```python
from build123d import *

# Parameters (mm, degrees)
SKETCH1_W           = 60
SKETCH1_H           = 35
SKETCH1_W_2         = 40.2
SKETCH1_H_2         = 20.2
BOSS_EXTRUDE1_DEPTH = 5
SKETCH2_W           = 60
SKETCH2_H           = 5
BOSS_EXTRUDE2_DEPTH = 29
SKETCH3_R           = 2
CUT_EXTRUDE1_DEPTH  = 10
SKETCH4_R           = 2
CUT_EXTRUDE2_DEPTH  = 48.451090489


with BuildPart() as part:
    # Sketch1 → Boss-Extrude1 (new body)
    with BuildSketch(Plane.XY):
        with Locations((-2.1, -1.998615043)):
            Rectangle(SKETCH1_W, SKETCH1_H)
        with Locations((-2.2, 0.601384957)):
            Rectangle(SKETCH1_W_2, SKETCH1_H_2, mode=Mode.SUBTRACT)
    extrude(amount=BOSS_EXTRUDE1_DEPTH)

    # Sketch2 → Boss-Extrude2 (add)
    with BuildSketch(Plane.XY.offset(5)):
        with Locations((-2.1, -16.998615043)):
            Rectangle(SKETCH2_W, SKETCH2_H)
    extrude(amount=BOSS_EXTRUDE2_DEPTH)

    # Sketch3 → Cut-Extrude1 (cut)
    with BuildSketch(Plane(origin=(0, -19.498615043, 0), x_dir=(-1, 0, 0), z_dir=(0, -1, 0))):
        with Locations(Location((17.1, -15, 0), (0, 0, 90))):
            Circle(SKETCH3_R)
        with Locations(Location((-12.9, -15, 0), (0, 0, 90))):
            Circle(SKETCH3_R)
    extrude(amount=-CUT_EXTRUDE1_DEPTH, mode=Mode.SUBTRACT)

    # Sketch4 → Cut-Extrude2 (cut, through all)
    with BuildSketch(Plane.XY.offset(5)):
        with Locations((21.9, 5.601384957)):
            Circle(SKETCH4_R)
        with Locations((21.9, -4.398615043)):
            Circle(SKETCH4_R)
        with Locations((-26.1, -4.398615043)):
            Circle(SKETCH4_R)
        with Locations((-26.1, 5.601384957)):
            Circle(SKETCH4_R)
    extrude(amount=-CUT_EXTRUDE2_DEPTH, mode=Mode.SUBTRACT)


solid = part.part
```
Build history of the part. All positions in model axes, mm. A direction names the side the tool comes from. Give positions to 0.01 mm unless a question says otherwise; leave off trailing zeros. Order: outer loops, then holes, each group sorted by start corner. A loop starts at its lowest first (then second) coordinate and runs counter-clockwise, first axis right, second up. Notation, with made-up numbers: M 21.25,57 L 46.25,57 A32 ccw 46.25,91 Z; hole C 31,89.5 d10. An arc over 180 degrees is marked long. Write item = value, one per line. Start each with the question number.
(1) Slice it at B-B on z = 15. Write the cut outline in (x, y), plus the area to 3 significant figures.
(2) Two-plate mould, pull along Y, no slides. Class faces 4 (the cylindrical face through (10.948, -17.034, 15.434)), 5 (the flat face through (-3, -19.499, 17)), 6 (the flat face through (-3, -14.499, 19)), 7 (the flat face through (-2, 10.701, 2)): released by +Y, released by -Y, zero draft, split by the parting line, or undercut.
(3) Slice it at C-C on y = -7.5. Write the cut outline in (x, z), plus the area to 3 significant figures.
(4) Slice it at A-A on x = 12.9. Write the cut outline in (y, z), plus the area to 3 significant figures.
(5) Slice it at D-D on x = -20. Write the cut outline in (y, z), plus the area to 3 significant figures.
(6) Pin check, flat tips, straight feed: pin 1 Ø6 at (x, y) = (14, -3) entering from +Z; pin 2 Ø4 at (x, z) = (-25.5, 29) entering from +Y; pin 3 Ø15 at (x, y) = (7, -3) entering from +Z. Stop position of each tip, or through.
(7) Probe L1, parallel to X at y = -17.95, z = 15; L2, parallel to Y at x = -26.1, z = 2.75; L3, parallel to X at y = 5.5, z = 4. List the from-to ranges inside material, lowest first. Write a range as [from, to].
(8) Which spindle directions (+Z, -Z, +X, -X, +Y, -Y) get a long thin tool onto all of the face, cutting with end or side? Do faces 1 (the flat face through (-3, 11, 5)), 2 (the cylindrical face through (-15.117, -17.034, 15.26)), 3 (the flat face through (17.9, 0, 2)). Say none if no direction does.
Responses:
q1.outline = M -32.1,-19.5 L -19.1,-19.5 L -19.1,-14.5 L -32.1,-14.5 Z; M -15.1,-19.5 L 10.9,-19.5 L 10.9,-14.5 L -15.1,-14.5 Z; M 14.9,-19.5 L 27.9,-19.5 L 27.9,-14.5 L 14.9,-14.5 Z
q1.area = 260 mm2
q2.face_4 = zero draft
q2.face_5 = released by -Y
q2.face_6 = released by +Y
q2.face_7 = undercut
q3.outline = M -32.1,0 L -22.3,0 L -22.3,5 L -32.1,5 Z; M 17.9,0 L 27.9,0 L 27.9,5 L 17.9,5 Z
q3.area = 99.0 mm2
q4.outline = M -19.5,0 L -9.5,0 L -9.5,5 L -14.5,5 L -14.5,13 L -19.5,13 Z; M -19.5,17 L -14.5,17 L -14.5,34 L -19.5,34 Z; M 10.7,0 L 15.5,0 L 15.5,5 L 10.7,5 Z
q4.area = 199 mm2
q5.outline = M -19.5,0 L -9.5,0 L -9.5,5 L -14.5,5 L -14.5,34 L -19.5,34 Z; M 10.7,0 L 15.5,0 L 15.5,5 L 10.7,5 Z
q5.area = 219 mm2
q6.pin_1 = through
q6.pin_2 = -14.5
q6.pin_3 = 5
q7.L1 = [-32.1, -19.1], [-15.1, 10.9], [14.9, 27.9]
q7.L2 = [-19.5, -6.4], [-2.4, 3.6], [7.6, 15.5]
q7.L3 = [-32.1, -28.1], [-24.1, -22.3], [17.9, 19.9], [23.9, 27.9]
q8.face_1 = +Z, +X, -X, +Y
q8.face_2 = +Y, -Y
q8.face_3 = +Z, -Z
